from build123d import *

# Parameters (mm, degrees)
SKETCH_1_W          = 45.9
SKETCH_1_H          = 38
EXTRUDE_1_DEPTH     = 3
CUT_EXTRUDE_3_DEPTH = 3.4
CUT_EXTRUDE_4_DEPTH = 3.4
CUT_EXTRUDE_5_DEPTH = 3
CUT_EXTRUDE_6_DEPTH = 3
SKETCH_9_R          = 2.5
CUT_EXTRUDE_7_DEPTH = 60.664143336


with BuildPart() as part:
    # 草图1 → 凸台-拉伸1 (new body)
    with BuildSketch(Plane.XY):
        with Locations((22.95, -19)):
            Rectangle(SKETCH_1_W, SKETCH_1_H)
    extrude(amount=EXTRUDE_1_DEPTH)

    # 草图3 → 切除-拉伸3 (cut)
    with BuildSketch(Plane.ZY):
        Polygon((3, -8.4), (3, -7.1), (0, -6.15), (0, -9.35), align=None)
        Polygon((0, -4.85), (3, -3.9), (3, 0), (0, 0), align=None)
        Polygon((3, -12.9), (3, -11.6), (0, -10.65), (0, -13.85), align=None)
        Polygon((3, -17.4), (3, -16.1), (0, -15.15), (0, -18.35), align=None)
        Polygon((3, -21.9), (3, -20.6), (0, -19.65), (0, -22.85), align=None)
        Polygon((3, -26.4), (3, -25.1), (0, -24.15), (0, -27.35), align=None)
        Polygon((3, -30.9), (3, -29.6), (0, -28.65), (0, -31.85), align=None)
        Polygon((3, -34.1), (0, -33.15), (0, -38), (3, -38), align=None)
    extrude(amount=-CUT_EXTRUDE_3_DEPTH, mode=Mode.SUBTRACT)

    # 草图5 → 切除-拉伸4 (cut)
    with BuildSketch(Plane(origin=(45.9, 0, 0), x_dir=(0, 0, -1), z_dir=(1, 0, 0))):
        Polygon((0, 0), (-3.00280668, 0), (-3.00280668, -3.9), (0, -4.85), align=None)
        Polygon((0, -6.15), (-3, -7.1), (-3, -8.4), (0, -9.35), align=None)
        Polygon((0, -33.15), (-3, -34.1), (-3, -38), (0, -38), align=None)
        Polygon((-3, -12.9), (0, -13.85), (0, -10.65), (-3, -11.6), align=None)
        Polygon((-3, -17.4), (0, -18.35), (0, -15.15), (-3, -16.1), align=None)
        Polygon((-3, -21.9), (0, -22.85), (0, -19.65), (-3, -20.6), align=None)
        Polygon((-3, -26.4), (0, -27.35), (0, -24.15), (-3, -25.1), align=None)
        Polygon((-3, -30.9), (0, -31.85), (0, -28.65), (-3, -29.6), align=None)
    extrude(amount=-CUT_EXTRUDE_4_DEPTH, mode=Mode.SUBTRACT)

    # 草图7 → 切除-拉伸5 (cut)
    with BuildSketch(Plane.XZ.offset(38)):
        Polygon((5.6, 3), (8.8, 3), (7.85, 0), (6.55, 0), align=None)
        Polygon((4.3, 3), (3.35, 0), (0, 0), (0, 3), align=None)
        Polygon((11.05, 0), (10.1, 3), (13.3, 3), (12.35, 0), align=None)
        Polygon((15.55, 0), (14.6, 3), (17.8, 3), (16.85, 0), align=None)
        Polygon((20.05, 0), (19.1, 3), (22.3, 3), (21.35, 0), align=None)
        Polygon((24.55, 0), (23.6, 3), (26.8, 3), (25.85, 0), align=None)
        Polygon((29.05, 0), (28.1, 3), (31.3, 3), (30.35, 0), align=None)
        Polygon((33.55, 0), (32.6, 3), (35.8, 3), (34.85, 0), align=None)
        Polygon((38.05, 0), (37.1, 3), (40.3, 3), (39.35, 0), align=None)
        Polygon((45.9, 0), (45.9, 3), (41.6, 3), (42.55, 0), align=None)
    extrude(amount=-CUT_EXTRUDE_5_DEPTH, mode=Mode.SUBTRACT)

    # 草图8 → 切除-拉伸6 (cut)
    with BuildSketch(Plane(origin=(0, 0, 0), x_dir=(1, 0, 0), z_dir=(0, 1, 0))):
        Polygon((6.55, 0), (5.6, -3), (8.8, -3), (7.85, 0), align=None)
        Polygon((3.35, 0), (4.3, -3), (0, -3), (0, 0), align=None)
        Polygon((12.35, 0), (11.05, 0), (10.1, -3), (13.3, -3), align=None)
        Polygon((16.85, 0), (15.55, 0), (14.6, -3), (17.8, -3), align=None)
        Polygon((21.35, 0), (20.05, 0), (19.1, -3), (22.3, -3), align=None)
        Polygon((25.85, 0), (24.55, 0), (23.6, -3), (26.8, -3), align=None)
        Polygon((30.35, 0), (29.05, 0), (28.1, -3), (31.3, -3), align=None)
        Polygon((34.85, 0), (33.55, 0), (32.6, -3), (35.8, -3), align=None)
        Polygon((39.35, 0), (38.05, 0), (37.1, -3), (40.3, -3), align=None)
        Polygon((45.9, -3), (45.9, 0), (42.55, 0), (41.6, -3), align=None)
    extrude(amount=-CUT_EXTRUDE_6_DEPTH, mode=Mode.SUBTRACT)

    # 草图9 → 切除-拉伸7 (cut, through all)
    with BuildSketch(Plane.XY.offset(3)):
        with Locations((32.4, -24.5)):
            Circle(SKETCH_9_R)
        with Locations((39.4, -29.5)):
            Circle(SKETCH_9_R)
        with Locations((6.5, -24.5)):
            Circle(SKETCH_9_R)
        with Locations((13.5, -29.5)):
            Circle(SKETCH_9_R)
        with BuildLine():
            Line((30.050510257, -16.5), (23.050510257, -16.5))
            ThreePointArc((23.050510257, -16.5), (20.550510257, -14), (23.050510257, -11.5))
            Line((23.050510257, -11.5), (30.050510257, -11.5))
            ThreePointArc((30.050510257, -11.5), (36, -14), (30.050510257, -16.5))
        make_face()
    extrude(amount=-CUT_EXTRUDE_7_DEPTH, mode=Mode.SUBTRACT)


solid = part.part
Verification items for the finished model (mm, model axes). A direction names the side the tool comes from. Give positions to 0.01 mm unless a question says otherwise; leave off trailing zeros. Answer as a JSON object with one key per item and string values. Group by question number.
1) Cross-section at A-A (z = 2.4). Give the number of separate pieces and of enclosed holes in the cut face, then the cut area to 3 significant figures.
2) Scan lines: line 1 along X through (y, z) = (-30.5, 1.8); line 2 along Y through (x, z) = (32.4, 1.8); line 3 along X through (y, z) = (-30, 2). Record each from-to range of solid material in increasing order. Write a range as [from, to].
3) Access from +Z, -Z, +X, -X, +Y, -Y to the whole of each face (thin tool, end or side, straight path). Record for faces 5 (the face through (42.044, -36.521, 1.599)), 6 (the face through (44.22, -17.87, 1.52)), 7 (the face through (6.08, -36.52, 1.48)).
4) Depth check by flat-ended pin: pin 1 Ø5 at (x, y) = (7, -30) entering from -Z; pin 2 Ø0.9 at (y, z) = (-30, 2) entering from +X. Enter the tip coordinate at first touch or a pass-through.
5) Mould release check, pull along X, two halves, no side actions. Record for faces 1 (the face through (0, -19, 2)), 2 (the face through (33.08, -36.52, 1.48)), 3 (the face through (44.22, -15.62, 1.48)), 4 (the face through (45.9, -19, 2)): released by +X, released by -X, zero draft, split by the parting line, or undercut.
Result sheet:
{
 "1": {"separate pieces": "1", "enclosed holes": "5", "area": "1,320 mm2"},
 "2": {"line 1": "x = [3.4, 11.21], [15.79, 37.11], [41.69, 42.5]", "line 2": "y = [-38, -27], [-22, -17.5], [-10.5, 0]", "line 3": "x = [3.4, 11.05], [15.95, 36.95], [41.85, 42.5]"},
 "3": {"face 5": "+Z, +X, -Y", "face 6": "-Z, +X", "face 7": "+Z, -Y"},
 "4": {"pin 1": "stops at z = 0", "pin 2": "stops at x = 42.5"},
 "5": {"face 1": "released by -X", "face 2": "undercut", "face 3": "zero draft", "face 4": "released by +X"}
}
